Part model, mm, in its own coordinate system. A direction names the side the tool comes from. Round coordinates to 2 decimals unless told otherwise and drop trailing zeros. Loops run counter-clockwise (first coordinate to the right, second up) from the corner with the lowest first, then second, coordinate; pieces in that order, holes last.
(1) Cut at A-A on y = 16.5. List the corners of the cut face in (x, z), then the cut area to 3 significant figures.
(2) Tool access for faces 4 (the face through (-18, 11, 8)), 5 (the face through (-26.5, -26.07, 7.6)): list every direction of +Z, -Z, +X, -X, +Y, -Y with a clear straight run to the whole face (end or side of a thin tool).
(3) Probe probe 1 along X at (y, z) = (6.5, 11.5); probe 2 along X at (y, z) = (-2, 12); probe 3 along Y at (x, z) = (-5, 11.25). List the from-to ranges inside material, lowest first.
(4) Mould opens along X. For faces 1 (the face through (26.5, -26.07, 7.6)), 2 (the face through (-28, 0, 8)), 3 (the face through (0, -18, 8)) say: +X half, -X half, draft (parallel to the pull), parting line (faces both ways), or undercut.
(5) Cut at C-C on x = 0. List the corners of the cut face in (y, z), then the cut area to 4 significant figures.
(6) Cut at D-D on x = -11. List the corners of the cut face in (y, z).
(7) Flat gauge pins, fed straight in: pin 1 (10 mm diameter, centred on x = -11, y = 13.5, fed in from +Z); pin 2 (4 mm diameter, centred on x = 2, z = 11.5, fed in from +Y). Where does each tip first touch, or does it go through?
from build123d import *

# Parameters (mm, degrees)
F1_DEPTH = 25
F2_R     = 4.99999
F3_DEPTH = 15
F4_DEPTH = 10


# Not quite as in the source:
# - a fillet or chamfer is up to 0.001 mm smaller than in the source, because OpenCascade refuses the exact size


with BuildPart() as f1:
    # F0 (on Top) → F1 (new body)
    with BuildSketch(Plane.XY):
        with BuildLine():
            Line((-28, -27.5), (28, -27.5))
            Line((28, -27.5), (28, 27.5))
            Line((28, 27.5), (18, 27.5))
            Line((18, 27.5), (18, 0))
            ThreePointArc((18, 0), (0, -18), (-18, 0))
            Line((-18, 0), (-18, 27.5))
            Line((-18, 27.5), (-28, 27.5))
            Line((-28, 27.5), (-28, -27.5))
        make_face()
    extrude(amount=F1_DEPTH)

    # F2 (radius 5 in the source; OpenCascade refuses exactly that, so slightly less here)
    f2_edges = [f1.edges().sort_by_distance(p)[0] for p in [
        (18, 27.5, 12.5),
        (-18, 27.5, 12.5),
        (28, 27.5, 12.5),
        (-28, 27.5, 12.5),
        (-28, -27.5, 12.5),
        (28, -27.5, 12.5),
    ]]
    fillet(f2_edges, radius=F2_R)

    # F3 (add): a face of the model
    f3_faces = [f1.faces().sort_by_distance(p)[0] for p in [
        (0, -26.7150796219, 25),
    ]]
    extrude(f3_faces, amount=-F3_DEPTH)

    # F4 (cut): a face of the model
    f4_faces = [f1.faces().sort_by_distance(p)[0] for p in [
        (0, -26.7150796219, 25),
    ]]
    extrude(f4_faces, amount=-F4_DEPTH, mode=Mode.SUBTRACT)


solid = f1.part
Final values:
1. outline: (-28, 0) - (-18, 0) - (-18, 15) - (-28, 15) - close; (18, 0) - (28, 0) - (28, 15) - (18, 15) - close
1. area: 300 mm2
2. face 4: +Z, -Z, +Y
2. face 5: +Z, -Z, -X, -Y
3. probe 1: x = -28 to -18, 18 to 28
3. probe 2: x = -28 to -17.89, 17.89 to 28
3. probe 3: y = -27.5 to -17.29
4. face 1: +X half
4. face 2: -X half
4. face 3: undercut
5. outline: (-27.5, 0) - (-18, 0) - (-18, 15) - (-27.5, 15) - close
5. area: 142.5 mm2
6. outline: (-27.5, 0) - (-14.25, 0) - (-14.25, 15) - (-27.5, 15) - close
7. pin 1: passes through
7. pin 2: stops at y = -17.55
